Here's how the part is built. I have some questions about the finished solid (model axes, mm). Face numbers are marked on the shaded views. A direction names the side the tool comes from. Coordinates: 2 decimals unless noted, no trailing zeros. Write each loop counter-clockwise with the first axis right and the second up, starting at its lowest first coordinate (ties: lowest second). Pieces come first, ordered by that corner, then holes.
Item 1: If we section it at C-C (y = -42.5): Please give me the cut outline in (x, z).
Item 2: If we section it at A-A (x = 0): Please give me the cut outline in (y, z), then the cut area to 3 significant figures.
Item 3: If I drill on line 1 (Z direction, x = 21, y = -19); line 2 (Z direction, x = -8, y = -35.5); line 3 (X direction, y = -22, z = 3), over which ranges is the centre line in solid material (lowest first)?
Item 4: I'm going to push flat-ended pins straight in: pin 1 Ø2.5 at (y, z) = (-44, 0.5) entering from -X; pin 2 Ø6 at (x, y) = (15.5, -17.5) entering from +Z; pin 3 Ø2 at (y, z) = (-31.5, 0.5) entering from +X; pin 4 Ø1.5 at (y, z) = (-41.5, 0.5) entering from +X. Where does each tip first touch, or does it pass through?
Item 5: For the marked faces 1 and 2, which set-ups out of +Z, -Z, +X, -X, +Y, -Y let a thin tool reach every point of the face, with its end or its side?
Item 6: If we section it at B-B (y = -5): Please give me the cut outline in (x, z), then the cut area to 3 significant figures.
Item 7: If we section it at D-D (x = -10): Please give me the cut outline in (y, z), then the cut area to 3 significant figures.
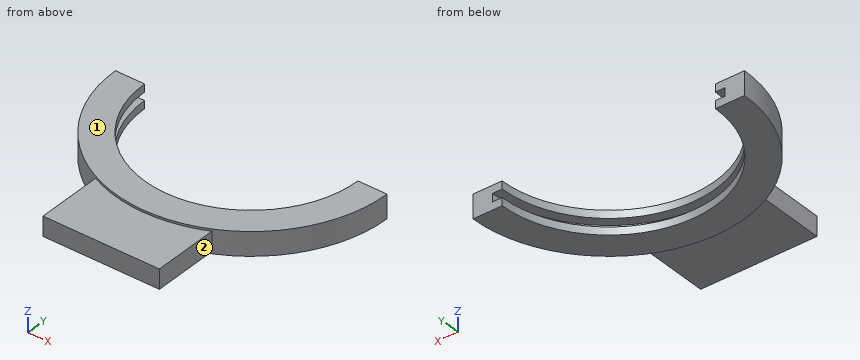
from build123d import *

# Parameters (mm, degrees)
F1_DEPTH = 1.05
F3_DEPTH = 2
F5_DEPTH = 2
F7_DEPTH = 2.5


with BuildPart() as f1:
    # F0 (on Top) → F1 (new body, symmetric)
    with BuildSketch(Plane.XY):
        with BuildLine():
            Line((35, 0), (30, 0))
            ThreePointArc((30, 0), (0, -30), (-30, 0))
            Line((-30, 0), (-35, 0))
            ThreePointArc((-35, 0), (0, -35), (35, 0))
        make_face()
    extrude(amount=F1_DEPTH, both=True)

    # F2 (on face) → F3 (join)
    with BuildSketch(Plane.XY.offset(1.05)):
        with BuildLine():
            ThreePointArc((-30, 0), (0, -30), (30, 0))
            Line((30, 0), (27.5, 0))
            ThreePointArc((27.5, 0), (0, -27.5), (-27.5, 0))
            Line((-27.5, 0), (-30, 0))
        make_face()
        with BuildLine():
            ThreePointArc((-35, 0), (0, -35), (35, 0))
            Line((35, 0), (30, 0))
            ThreePointArc((30, 0), (0, -30), (-30, 0))
            Line((-30, 0), (-35, 0))
        make_face()
    extrude(amount=F3_DEPTH)

    # F4 (on face) → F5 (join)
    with BuildSketch(Plane(origin=(0, 0, -1.05), x_dir=(1, 0, 0), z_dir=(0, 0, -1))):
        with BuildLine():
            Line((30, 0), (35, 0))
            ThreePointArc((35, 0), (0, 35), (-35, 0))
            Line((-35, 0), (-30, 0))
            ThreePointArc((-30, 0), (0, 30), (30, 0))
        make_face()
        with BuildLine():
            Line((27.5, 0), (30, 0))
            ThreePointArc((30, 0), (0, 30), (-30, 0))
            Line((-30, 0), (-27.5, 0))
            ThreePointArc((-27.5, 0), (0, 27.5), (27.5, 0))
        make_face()
    extrude(amount=F5_DEPTH)

    # F6 (on Top) → F7 (join, symmetric)
    with BuildSketch(Plane.XY):
        with BuildLine():
            Line((0, -48.6514897645), (0, -33.6514897645))
            ThreePointArc((0, -33.6514897645), (-7.624504365, -32.7740115893), (-15, -30.6514897645))
            Line((-15, -30.6514897645), (-15, -48.6514897645))
            Line((-15, -48.6514897645), (0, -48.6514897645))
        make_face()
        with BuildLine():
            ThreePointArc((15, -30.6514897645), (7.624504365, -32.7740115893), (0, -33.6514897645))
            Line((0, -33.6514897645), (0, -48.6514897645))
            Line((0, -48.6514897645), (15, -48.6514897645))
            Line((15, -48.6514897645), (15, -30.6514897645))
        make_face()
    extrude(amount=F7_DEPTH, both=True)


solid = f1.part
Answer list:
1. outline: (-15, -2.5) - (15, -2.5) - (15, 2.5) - (-15, 2.5) - close
2. outline: (-48.65, -2.5) - (-35, -2.5) - (-35, -3.05) - (-27.5, -3.05) - (-27.5, -1.05) - (-30, -1.05) - (-30, 1.05) - (-27.5, 1.05) - (-27.5, 3.05) - (-35, 3.05) - (-35, 2.5) - (-48.65, 2.5) - close
2. area: 109 mm2
3. line 1: z = -3.05 to -1.05, 1.05 to 3.05
3. line 2: z = -2.5 to 2.5
3. line 3: x = -27.22 to -16.5, 16.5 to 27.22
4. pin 1: stops at x = -15
4. pin 2: passes through
4. pin 3: stops at x = 17.17
4. pin 4: stops at x = 15
5. face 1: +Z, +X, -X, +Y, -Y
5. face 2: +Z, -Z, +X, -Y
6. outline: (-34.64, -3.05) - (-27.04, -3.05) - (-27.04, -1.05) - (-29.58, -1.05) - (-29.58, 1.05) - (-27.04, 1.05) - (-27.04, 3.05) - (-34.64, 3.05) - close; (27.04, -3.05) - (34.64, -3.05) - (34.64, 3.05) - (27.04, 3.05) - (27.04, 1.05) - (29.58, 1.05) - (29.58, -1.05) - (27.04, -1.05) - close
6. area: 82.0 mm2
7. outline: (-48.65, -2.5) - (-33.54, -2.5) - (-33.54, -3.05) - (-25.62, -3.05) - (-25.62, -1.05) - (-28.28, -1.05) - (-28.28, 1.05) - (-25.62, 1.05) - (-25.62, 3.05) - (-33.54, 3.05) - (-33.54, 2.5) - (-48.65, 2.5) - close
7. area: 118 mm2
